Source: CAD feature listing. Evaluate the final solid. Frame: model axes, mm. Face numbers are marked on the shaded views. A direction names the side the tool comes from. Round coordinates to 2 decimals unless told otherwise and drop trailing zeros. Write each loop counter-clockwise with the first axis right and the second up, starting at its lowest first coordinate (ties: lowest second). Pieces come first, ordered by that corner, then holes. Notation, with made-up numbers: M 23,17 L 80,17 A27 cw 80,34 Z; hole C 82.5,53.25 d7. An arc over 180 degrees is marked long. Answer in a Markdown table with one row per item.
from build123d import *

# Parameters (mm, degrees)
SKICA2_W                 = 20
SKICA2_H                 = 42.3
P_IDAT_VYSUNUT_M1_DEPTH  = 4
SKICA3_W                 = 24
SKICA3_H                 = 42.3
P_IDAT_VYSUNUT_M2_DEPTH  = 4
SKICA4_W                 = 6
SKICA4_H                 = 42.3
P_IDAT_VYSUNUT_M3_DEPTH  = 42.3
SKICA5_R                 = 11.05
ODEBRAT_VYSUNUT_M1_DEPTH = 7
SKICA7_R                 = 2.6
ODEBRAT_VYSUNUT_M3_DEPTH = 4
ZKOSEN_1_SIZE            = 1
SKICA8_W                 = 20
SKICA8_H                 = 4
P_IDAT_VYSUNUT_M4_DEPTH  = 20.091596743
SKICA9_R                 = 2.6
ODEBRAT_VYSUNUT_M4_DEPTH = 4
ODEBRAT_VYSUNUT_M5_DEPTH = 80
SKICA11_W                = 6
SKICA11_H                = 6
SKICA11_H_2              = 10
P_IDAT_VYSUNUT_M5_DEPTH  = 8
SKICA13_R                = 1.6
ODEBRAT_VYSUNUT_M6_DEPTH = 15
SKICA14_W                = 5
SKICA14_H                = 3
ODEBRAT_VYSUNUT_M7_DEPTH = 15
ZKOSEN_2_SIZE            = 1


with BuildPart() as part:
    # Skica2 → Přidat vysunutím1 (new body)
    with BuildSketch(Plane.XY):
        with Locations((-14.524287798, -61.15)):
            Rectangle(SKICA2_W, SKICA2_H)
    extrude(amount=P_IDAT_VYSUNUT_M1_DEPTH)

    # Skica3 → Přidat vysunutím2 (add)
    with BuildSketch(Plane.ZY.offset(24.524287798)):
        with Locations((-8, -61.15)):
            Rectangle(SKICA3_W, SKICA3_H)
    extrude(amount=P_IDAT_VYSUNUT_M2_DEPTH)

    # Skica4 → Přidat vysunutím3 (add)
    with BuildSketch(Plane.XY.offset(4)):
        with Locations((-7.524287798, -61.15)):
            Rectangle(SKICA4_W, SKICA4_H)
    extrude(amount=P_IDAT_VYSUNUT_M3_DEPTH)

    # Skica5 → Odebrat vysunutím1 (cut)
    with BuildSketch(Plane(origin=(-4.524287798, 0, 0), x_dir=(0, 0, -1), z_dir=(1, 0, 0))):
        with Locations((-25.15, -61.15)):
            Circle(SKICA5_R)
    extrude(amount=-ODEBRAT_VYSUNUT_M1_DEPTH, mode=Mode.SUBTRACT)

    # Skica7 → Odebrat vysunutím3 (cut)
    with BuildSketch(Plane.ZY.offset(28.524287798)):
        with Locations(Location((-10, -50, 0), (0, 0, 270))):
            Circle(SKICA7_R)
        with Locations(Location((-10, -70, 0), (0, 0, 270))):
            Circle(SKICA7_R)
    extrude(amount=-ODEBRAT_VYSUNUT_M3_DEPTH, mode=Mode.SUBTRACT)

    # Zkosení1
    zkosen_1_edges = [part.edges().sort_by_distance(p)[0] for p in [
        (-10.524287798, -61.15, 36.2),
    ]]
    chamfer(zkosen_1_edges, length=ZKOSEN_1_SIZE)

    # Skica8 → Přidat vysunutím4 (add)
    with BuildSketch(Plane.XZ.offset(82.3)):
        with Locations((-14.524287798, 2)):
            Rectangle(SKICA8_W, SKICA8_H)
    extrude(amount=P_IDAT_VYSUNUT_M4_DEPTH)

    # Skica9 → Odebrat vysunutím4 (cut)
    with BuildSketch(Plane.XY.offset(4)):
        with Locations((-14.524287798, -92.391596743)):
            Circle(SKICA9_R)
    extrude(amount=-ODEBRAT_VYSUNUT_M4_DEPTH, mode=Mode.SUBTRACT)

    # Skica10 → Odebrat vysunutím5 (cut)
    with BuildSketch(Plane.ZY.offset(10.524287798)):
        Polygon((46.3, -44), (42.3, -40), (46.565878614, -39.259270079), align=None)
        Polygon((42.3, -82.3), (46.3, -78.3), (47.745576453, -80.3), (46.3, -85.415433185), align=None)
    extrude(amount=-ODEBRAT_VYSUNUT_M5_DEPTH, mode=Mode.SUBTRACT)

    # Skica11 → Přidat vysunutím5 (add)
    with BuildSketch(Plane(origin=(0, -40, 0), x_dir=(1, 0, 0), z_dir=(0, 1, 0))):
        with Locations((-7.524287798, -39.3)):
            Rectangle(SKICA11_W, SKICA11_H)
        with Locations((-7.524287798, -19.3)):
            Rectangle(SKICA11_W, SKICA11_H_2)
    extrude(amount=P_IDAT_VYSUNUT_M5_DEPTH)

    # Skica13 → Odebrat vysunutím6 (cut)
    with BuildSketch(Plane(origin=(0, -32, 0), x_dir=(1, 0, 0), z_dir=(0, 1, 0))):
        with Locations(Location((-7.524287798, -39.3, 0), (0, 0, 270))):
            Circle(SKICA13_R)
        with Locations(Location((-7.524287798, -19.3, 0), (0, 0, 270))):
            Circle(SKICA13_R)
    extrude(amount=-ODEBRAT_VYSUNUT_M6_DEPTH, mode=Mode.SUBTRACT)

    # Skica14 → Odebrat vysunutím7 (cut)
    with BuildSketch(Plane(origin=(-4.524287798, 0, 0), x_dir=(0, 0, -1), z_dir=(1, 0, 0))):
        with Locations((-39.3, -44.438988808)):
            Rectangle(SKICA14_W, SKICA14_H)
        with Locations((-19.3, -44.438988808)):
            Rectangle(SKICA14_W, SKICA14_H)
    extrude(amount=-ODEBRAT_VYSUNUT_M7_DEPTH, mode=Mode.SUBTRACT)

    # Zkosení2
    zkosen_2_edges = [part.edges().sort_by_distance(p)[0] for p in [
        (-4.524287798, -61.15, 36.2),
    ]]
    chamfer(zkosen_2_edges, length=ZKOSEN_2_SIZE)


solid = part.part
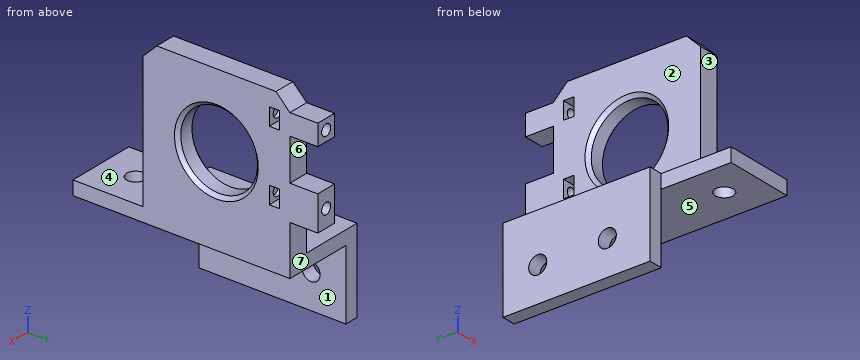
Q1. Pull-direction query (Z, two-part tool) for the marked faces 4, 5, 6 and 7; classes: pulls with the +Z half, pulls with the -Z half, needs draft (parallel to the pull), parting line crosses it, or undercut.
Solutions:
| item | result |
|---|---|
| face 4 | pulls with the +Z half |
| face 5 | pulls with the -Z half |
| face 6 | undercut |
| face 7 | needs draft |
Q2. Section C-C (z = 25.15). Return loops of the section in (x, y).
Solutions:
| item | result |
|---|---|
| outline | M -10.52,-82.3 L -4.52,-82.3 L -4.52,-73.2 L -5.52,-72.2 L -9.52,-72.2 L -10.52,-73.2 Z; M -10.52,-49.1 L -9.52,-50.1 L -5.52,-50.1 L -4.52,-49.1 L -4.52,-40 L -10.52,-40 Z |
Q3. Access query for the marked faces 1, 2 and 3. Directions: +Z, -Z, +X, -X, +Y, -Y. A direction counts if a zero-diameter tool reaches every point of the face in a straight line with its end or side. Return the directions, or none.
Solutions:
| item | result |
|---|---|
| face 1 | -Z, +X, +Y, -Y |
| face 2 | +Z, -X, +Y, -Y |
| face 3 | +Z, +X, -X, -Y |
Q4. Section A-A (z = -10). Return loops of the section in (x, y).
Solutions:
| item | result |
|---|---|
| outline | M -28.52,-82.3 L -24.52,-82.3 L -24.52,-72.6 L -28.52,-72.6 Z; M -28.52,-67.4 L -24.52,-67.4 L -24.52,-52.6 L -28.52,-52.6 Z; M -28.52,-47.4 L -24.52,-47.4 L -24.52,-40 L -28.52,-40 Z |
Q5. Material intervals for probe 1 along X at (y, z) = (-46.2, 39.3); probe 2 along Y at (x, z) = (-7.8, 25.15); probe 3 along Z at (x, y) = (-27.5, -70), sorted ascending.
Solutions:
| item | result |
|---|---|
| probe 1 | x = -10.52 to -9.12, -5.92 to -4.52 |
| probe 2 | y = -82.3 to -72.2, -50.1 to -40 |
| probe 3 | z = -20 to -12.6, -7.4 to 4 |
Q6. Section D-D (x = -13.5). Return loops of the section in (y, z), and give its area (3 significant figures).
Solutions:
| item | result |
|---|---|
| outline | M -102.39,0 L -94.78,0 L -94.78,4 L -102.39,4 Z; M -90,0 L -40,0 L -40,4 L -90,4 Z |
| area | 230 mm2 |
Q7. Contact query for flat-ended pins moving along their axis: pin 1 Ø3 at (x, z) = (-7.52, 39.3) entering from +Y; pin 2 Ø1.5 at (x, y) = (-21, -85.5) entering from -Z; pin 3 Ø6.5 at (x, y) = (-6.5, -35) entering from +Z; pin 4 Ø12 at (y, z) = (-59, 22.5) entering from -X. Output: stop coordinate, or through.
Solutions:
| item | result |
|---|---|
| pin 1 | stops at y = -47 |
| pin 2 | stops at z = 0 |
| pin 3 | stops at z = 42.3 |
| pin 4 | passes through |
Q8. Section B-B (y = -39). Return loops of the section in (x, z).
Solutions:
| item | result |
|---|---|
| outline | M -10.52,14.3 L -4.52,14.3 L -4.52,24.3 L -10.52,24.3 Z; M -10.52,36.3 L -4.52,36.3 L -4.52,42.3 L -10.52,42.3 Z; hole C -7.52,19.3 d3.2; hole C -7.52,39.3 d3.2 |
